```python
from build123d import *

# Parameters (mm, degrees)
SKETCH1_R           = 2.65
BOSS_EXTRUDE1_DEPTH = 10
SKETCH2_W           = 43
SKETCH2_H           = 24
BOSS_EXTRUDE2_DEPTH = 50
CHAMFER12_SIZE      = 25
SKETCH11_W          = 40.1
SKETCH11_H          = 21
CUT_EXTRUDE3_DEPTH  = 40
BOSS_EXTRUDE3_DEPTH = 43
FILLET1_R           = 10
FILLET5_R           = 1
CUT_EXTRUDE4_DEPTH  = 2


with BuildPart() as part:
    # Sketch1 → Boss-Extrude1 (new body)
    with BuildSketch(Plane(origin=(0, 0, 0), x_dir=(1, 0, 0), z_dir=(0, 1, 0))):
        Polygon((0, 0), (150, 0), (150, 62.5), (99, 62.5), (51, 62.5), (0, 62.5), align=None)
        with Locations(Location((108.05464, 46.5, 0), (0, 0, 270))):
            Circle(SKETCH1_R, mode=Mode.SUBTRACT)
        with Locations(Location((41.87366, 46.5, 0), (0, 0, 270))):
            Circle(SKETCH1_R, mode=Mode.SUBTRACT)
        with Locations(Location((41.87366, 16, 0), (0, 0, 270))):
            Circle(SKETCH1_R, mode=Mode.SUBTRACT)
        with Locations(Location((108.05464, 16, 0), (0, 0, 270))):
            Circle(SKETCH1_R, mode=Mode.SUBTRACT)
    extrude(amount=BOSS_EXTRUDE1_DEPTH)

    # Sketch2 → Boss-Extrude2 (add)
    with BuildSketch(Plane.XZ):
        with Locations((75, -31.5)):
            Rectangle(SKETCH2_W, SKETCH2_H)
    extrude(amount=BOSS_EXTRUDE2_DEPTH)

    # Chamfer12
    chamfer12_edges = [part.edges().sort_by_distance(p)[0] for p in [
        (53.5, 0, -31.5),
        (96.5, 0, -31.5),
    ]]
    chamfer(chamfer12_edges, length=CHAMFER12_SIZE)

    # Sketch11 → Cut-Extrude3 (cut)
    with BuildSketch(Plane.XZ.offset(50)):
        with Locations((75.00366, -31.5)):
            Rectangle(SKETCH11_W, SKETCH11_H)
    extrude(amount=-CUT_EXTRUDE3_DEPTH, mode=Mode.SUBTRACT)

    # Sketch12 → Boss-Extrude3 (add)
    with BuildSketch(Plane.ZY.offset(-53.5)):
        Polygon((-43.5, -25), (-43.5, 0), (-62.5, 0), align=None)
    extrude(amount=-BOSS_EXTRUDE3_DEPTH)

    # Fillet1
    fillet1_edges = [part.edges().sort_by_distance(p)[0] for p in [
        (28.5, 0, -31.5),
        (121.5, 0, -31.5),
    ]]
    fillet(fillet1_edges, radius=FILLET1_R)

    # Fillet5
    # the kernel refuses this fillet: 1 mm, written as the material it adds along each edge
    with BuildSketch(Plane(origin=(96.5, 0, -41), x_dir=(1, 0, 0), z_dir=(0, 0, -1))) as fillet5_piece_1_section:
        with BuildLine():
            CenterArc((FILLET5_R, FILLET5_R), FILLET5_R, 180, 90)
            Line((0, FILLET5_R), (0, 0))
            Line((0, 0), (FILLET5_R, 0))
        make_face()
    fillet5_piece_1 = extrude(amount=21.5, mode=Mode.PRIVATE)
    fillet5_piece_1 = split(fillet5_piece_1, bisect_by=Plane(origin=(96.726395114, -9.898830574, -54.976888763), z_dir=(0, 0.6050832675335575, 0.7961621941231029)), keep=Keep.TOP, mode=Mode.PRIVATE)
    add(fillet5_piece_1)
    with BuildSketch(Plane(origin=(96.5, -27.5, -43.5), x_dir=(1, 0, 0), z_dir=(0, 1, 0))) as fillet5_piece_2_section:
        with BuildLine():
            CenterArc((FILLET5_R, FILLET5_R), FILLET5_R, 180, 90)
            Line((0, FILLET5_R), (0, 0))
            Line((0, 0), (FILLET5_R, 0))
        make_face()
    fillet5_piece_2 = extrude(amount=30, mode=Mode.PRIVATE)
    fillet5_piece_2 = split(fillet5_piece_2, bisect_by=Plane(origin=(102.972342409, -18.527657591, -43.72500317), z_dir=(-0.7071067811865476, 0.7071067811865476, 0)), keep=Keep.TOP, mode=Mode.PRIVATE)
    fillet5_piece_2 = split(fillet5_piece_2, bisect_by=Plane(origin=(96.726036712, -16.829582585, -49.709517236), z_dir=(0, 0.6050832675335575, 0.7961621941231029)), keep=Keep.TOP, mode=Mode.PRIVATE)
    add(fillet5_piece_2)
    with BuildSketch(Plane(origin=(53.5, 0, -41), x_dir=(-1, 0, 0), z_dir=(0, 0, -1))) as fillet5_piece_3_section:
        with BuildLine():
            CenterArc((FILLET5_R, -FILLET5_R), FILLET5_R, 90, 90)
            Line((0, -FILLET5_R), (0, 0))
            Line((0, 0), (FILLET5_R, 0))
        make_face()
    fillet5_piece_3 = extrude(amount=21.5, mode=Mode.PRIVATE)
    fillet5_piece_3 = split(fillet5_piece_3, bisect_by=Plane(origin=(53.273604886, -9.898830574, -54.976888763), z_dir=(0, 0.6050832675335575, 0.7961621941231029)), keep=Keep.TOP, mode=Mode.PRIVATE)
    add(fillet5_piece_3)
    with BuildSketch(Plane(origin=(53.5, -27.5, -43.5), x_dir=(0, 0, -1), z_dir=(0, 1, 0))) as fillet5_piece_4_section:
        with BuildLine():
            CenterArc((FILLET5_R, FILLET5_R), FILLET5_R, 180, 90)
            Line((0, FILLET5_R), (0, 0))
            Line((0, 0), (FILLET5_R, 0))
        make_face()
    fillet5_piece_4 = extrude(amount=30, mode=Mode.PRIVATE)
    fillet5_piece_4 = split(fillet5_piece_4, bisect_by=Plane(origin=(47.02765759, -18.52765759, -43.72500317), z_dir=(0.7071067811865476, 0.7071067811865476, 0)), keep=Keep.TOP, mode=Mode.PRIVATE)
    fillet5_piece_4 = split(fillet5_piece_4, bisect_by=Plane(origin=(53.273963288, -16.829582583, -49.709517237), z_dir=(0, 0.6050832675335575, 0.7961621941231029)), keep=Keep.TOP, mode=Mode.PRIVATE)
    add(fillet5_piece_4)

    # Sketch14 → Cut-Extrude4 (cut)
    with BuildSketch(Plane(origin=(0, 0, -43.5), x_dir=(-1, 0, 0), z_dir=(0, 0, -1))):
        with BuildLine():
            Line((-24.357864376, 0), (-52.5, 0))
            Line((-52.5, 0), (-52.5, -24))
            Line((-52.5, -24), (-31.428932188, -2.928932188))
            ThreePointArc((-31.428932188, -2.928932188), (-28.1846987, -0.761204675), (-24.357864376, 0))
        make_face()
        with BuildLine():
            Line((-97.5, -24), (-97.5, 0))
            Line((-97.5, 0), (-125.642135624, 0))
            ThreePointArc((-125.642135624, 0), (-121.8153013, -0.761204675), (-118.571067812, -2.928932188))
            Line((-118.571067812, -2.928932188), (-97.5, -24))
        make_face()
    extrude(amount=-CUT_EXTRUDE4_DEPTH, mode=Mode.SUBTRACT)


solid = part.part
```
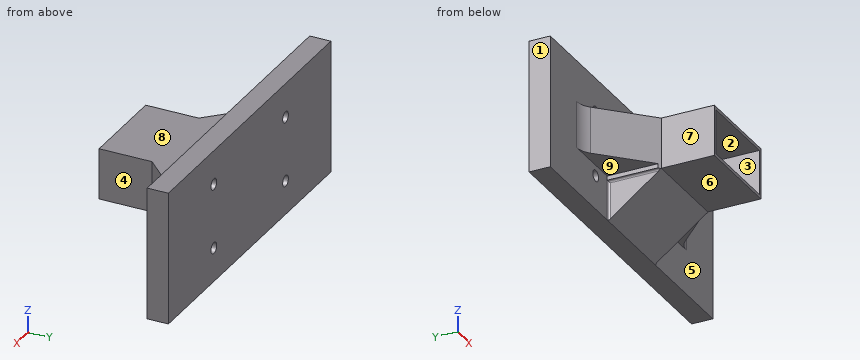
Could you check a few things on this model? Use its own coordinates, in mm. Face numbers are marked on the shaded views. A direction names the side the tool comes from. Round coordinates to 2 decimals unless told otherwise and drop trailing zeros. Loops run counter-clockwise (first coordinate to the right, second up) from the corner with the lowest first, then second, coordinate; pieces in that order, holes last. Notation, with made-up numbers: (-19.5, 69) - (32.5, 69) arc R20 cw to (32.5, 89) - close; hole circle Ø7 at (63, -7.75). An arc over 180 degrees is marked (long way). Answer in a Markdown table with one row per item. Add a question column.
(1) I need wall thicknesses on line 1 along X through (y, z) = (6.25, -46.5); line 2 along Z through (x, y) = (67, -28); line 3 along Y through (x, z) = (124.5, -3). Which ranges of each line are inside material? Lowest first, please.
(2) If we section it at D-D (y = -21.5): Please give me the cut outline in (x, z).
(3) If we mould it in two halves opening along X, with no side actions, what happens to the marked faces 1, 2, 3 and 4? For each: pulls with the +X half, pulls with the -X half, needs draft (parallel to the pull), parting line crosses it, or undercut.
(4) If we section it at B-B (z = -16): Please give me the cut outline in (x, y).
(5) I'm going to push flat-ended pins straight in: pin 1 (1 mm diameter, centred on y = -14, z = -42.5, fed in from +X); pin 2 (19 mm diameter, centred on y = -16, z = -51.5, fed in from -X); pin 3 (17 mm diameter, centred on y = -32, z = -34.5, fed in from +X); pin 4 (1.5 mm diameter, centred on y = -35, z = -45.5, fed in from -X). Where does each tip first touch, or does it pass through?
(6) For the marked faces 5, 6, 7, 8 and 9, which set-ups out of +Z, -Z, +X, -X, +Y, -Y let a thin tool reach every point of the face, with its end or its side?
(7) If we section it at C-C (x = 34): Please give me the cut outline in (y, z), plus the area to 3 significant figures.
(8) If we section it at A-A (y = -38): Please give me the cut outline in (x, z), plus the area to 3 significant figures.
Model answer:
| question | item | result |
|---|---|---|
| 1 | line 1 | x = 0 to 39.22, 44.52 to 105.4, 110.7 to 150 |
| 1 | line 2 | z = -43.5 to -42, -21 to -19.5 |
| 1 | line 3 | y = 0 to 10 |
| 2 | outline | (50, -41.5) - (52.5, -41.5) - (52.5, -43.5) arc R1 cw to (53.5, -44.5) - (53.5, -46.16) - (96.5, -46.16) - (96.5, -44.5) arc R1 cw to (97.5, -43.5) - (97.5, -41.5) - (100, -41.5) - (100, -19.5) - (50, -19.5) - close; hole (54.95, -42) - (95.05, -42) - (95.05, -21) - (54.95, -21) - close |
| 3 | face 1 | pulls with the -X half |
| 3 | face 2 | undercut |
| 3 | face 3 | undercut |
| 3 | face 4 | pulls with the +X half |
| 4 | outline | (0, 0) - (39.22, 0) - (39.22, 10) - (0, 10) - close; (44.52, 0) - (105.4, 0) - (105.4, 10) - (44.52, 10) - close; (110.7, 0) - (150, 0) - (150, 10) - (110.7, 10) - close |
| 5 | pin 1 | stops at x = 97.5 |
| 5 | pin 2 | stops at x = 52.5 |
| 5 | pin 3 | stops at x = 98 |
| 5 | pin 4 | passes through |
| 6 | face 5 | -Y |
| 6 | face 6 | -Z, +X, -X, -Y |
| 6 | face 7 | +Z, -Z, -X, -Y |
| 6 | face 8 | +Z, +X, -X, -Y |
| 6 | face 9 | -Z, -X, -Y |
| 7 | outline | (-5.5, -41.5) - (0, -41.5) - (0, -62.5) - (10, -62.5) - (10, 0) - (0, 0) - (0, -19.5) - (-5.5, -19.5) - close |
| 7 | area | 746 mm² |
| 8 | outline | (53.5, -43.5) - (96.5, -43.5) - (96.5, -19.5) - (53.5, -19.5) - close; hole (54.95, -42) - (95.05, -42) - (95.05, -21) - (54.95, -21) - close |
| 8 | area | 190 mm² |
